from build123d import *

# Parameters (mm, degrees)
SKETCH1_W           = 70
SKETCH1_H           = 25
SKETCH1_R           = 1.6
BOSS_EXTRUDE1_DEPTH = 10
BOSS_EXTRUDE2_DEPTH = 25
SKETCH3_R           = 3
CUT_EXTRUDE1_DEPTH  = 39.487010796
FILLET1_R           = 2
SKETCH6_R           = 1.6
CUT_EXTRUDE3_DEPTH  = 27
SKETCH7_W           = 2.6
SKETCH7_H           = 6
CUT_EXTRUDE4_DEPTH  = 11.25


with BuildPart() as part:
    # Sketch1 → Boss-Extrude1 (new body)
    with BuildSketch(Plane(origin=(0, 0, 0), x_dir=(1, 0, 0), z_dir=(0, 1, 0))):
        Rectangle(SKETCH1_W, SKETCH1_H)
        with Locations(Location((-26, -1, 0), (0, 0, 270))):
            Circle(SKETCH1_R, mode=Mode.SUBTRACT)
        with Locations(Location((26, -1, 0), (0, 0, 270))):
            Circle(SKETCH1_R, mode=Mode.SUBTRACT)
    extrude(amount=BOSS_EXTRUDE1_DEPTH)

    # Sketch2 → Boss-Extrude2 (add)
    with BuildSketch(Plane.XY.offset(12.5)):
        Polygon((-35, 0), (-20.773502692, 0), (-15, -10), (-35, -10), align=None)
        Polygon((35, 0), (35, -10), (15, -10), (20.773502692, 0), align=None)
    extrude(amount=-BOSS_EXTRUDE2_DEPTH)

    # Sketch3 → Cut-Extrude1 (cut, through all)
    with BuildSketch(Plane.XZ):
        with Locations(Location((-26, 1, 0), (0, 0, 270))):
            Circle(SKETCH3_R)
        with Locations(Location((26, 1, 0), (0, 0, 270))):
            Circle(SKETCH3_R)
    extrude(amount=CUT_EXTRUDE1_DEPTH, mode=Mode.SUBTRACT)

    # Fillet1
    fillet1_edges = [part.edges().sort_by_distance(p)[0] for p in [
        (35, 10, 0),
        (0, 10, -12.5),
        (0, 0, -12.5),
        (0, 0, 12.5),
        (-17.886751346, -5, -12.5),
        (-25, -10, -12.5),
        (-15, -10, 0),
        (-25, -10, 12.5),
        (-17.886751346, -5, 12.5),
        (25, -10, -12.5),
        (17.886751346, -5, -12.5),
        (15, -10, 0),
        (25, -10, 12.5),
        (17.886751346, -5, 12.5),
        (-35, 10, 0),
        (-35, 0, -12.5),
        (35, 0, -12.5),
        (35, 0, 12.5),
        (-35, 0, 12.5),
        (0, 10, 12.5),
    ]]
    fillet(fillet1_edges, radius=FILLET1_R)

    # Sketch6 → Cut-Extrude3 (cut)
    with BuildSketch(Plane.ZY.offset(35)):
        with Locations((-8.5, -4)):
            Circle(SKETCH6_R)
        with Locations((7.5, -4)):
            Circle(SKETCH6_R)
    extrude(amount=-CUT_EXTRUDE3_DEPTH, mode=Mode.SUBTRACT)

    # Sketch7 → Cut-Extrude4 (cut)
    with BuildSketch(Plane.XZ.offset(10)):
        with Locations((-30, -8.5)):
            Rectangle(SKETCH7_W, SKETCH7_H)
        with Locations((-30, 7.5)):
            Rectangle(SKETCH7_W, SKETCH7_H)
    extrude(amount=-CUT_EXTRUDE4_DEPTH, mode=Mode.SUBTRACT)


solid = part.part
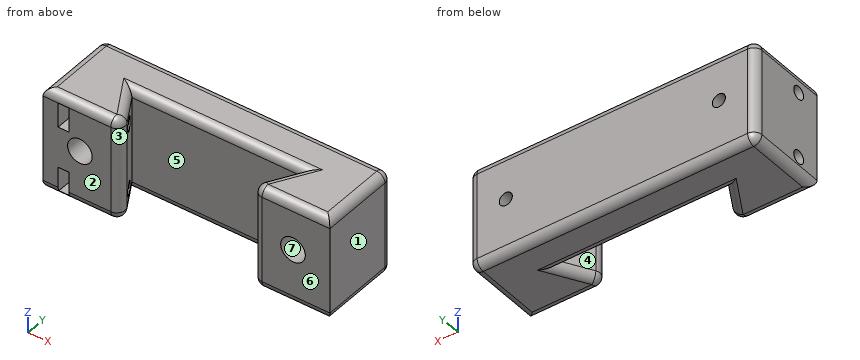
Can you work these out from the model? Positions are in its coordinate system, mm. Face numbers are marked on the shaded views. A direction names the side the tool comes from. Give positions to 0.01 mm unless a question says otherwise; leave off trailing zeros. Write each loop counter-clockwise with the first axis right and the second up, starting at its lowest first coordinate (ties: lowest second). Pieces come first, ordered by that corner, then holes. Notation, with made-up numbers: (53.5, 38) -> (95.5, 38) arc R8 cw to (95.5, 47) -> close; hole circle Ø3 at (25.25, 48). An arc over 180 degrees is marked (long way). Answer as a JSON object with one key per item and string values. Group by question number.
Item 1: I'm going to push flat-ended pins straight in: P1, Ø2, axis at x = -30, z = 6, coming from the -Y side; P2, Ø4, axis at x = 26, z = 1, coming from the -Y side; P3, Ø1.9, axis at y = -4, z = 7.5, coming from the -X side. Where does each tip first touch, or does it pass through?
Item 2: Please list where these lines run through material, in increasing order: line 1 (X direction, y = 4.5, z = 1); line 2 (Y direction, x = -32.65, z = -8.5); line 3 (X direction, y = -8.75, z = 9.5). Write a range as [from, to].
Item 3: Suppose I cut it at A-A (x = 26). Please give me the cut outline in (y, z), plus the area to 3 significant figures.
Item 4: For the marked faces 5, 6 and 7, which set-ups out of +Z, -Z, +X, -X, +Y, -Y let a thin tool reach every point of the face, with its end or its side?
Item 5: We'd pull the mould along Y, two halves only. Please class the marked faces 1, 2, 3 and 4: +Y half, -Y half, draft (parallel to the pull), parting line (faces both ways), or undercut.
Item 6: Suppose I cut it at D-D (x = -4.5). Please give me the cut outline in (y, z).
Item 7: Suppose I cut it at C-C (y = -4). State how many separate pieces and enclosed holes the cut face has, plus the area to 3 significant figures.
Item 8: Suppose I cut it at B-B (z = -8.5). Please give me the cut outline in (x, y).
Findings:
{
 "1": {"P1": "stops at y = 1.25", "P2": "stops at y = 0", "P3": "stops at x = 17.92"},
 "2": {"line 1": "x = [-35, -27.6], [-24.4, 24.4], [27.6, 35]", "line 2": "y = [-10, -5.6], [-2.4, 10]", "line 3": "x = [-35, -31.3], [-28.7, -16.61], [16.61, 35]"},
 "3": {"outline": "(-10, -10.5) arc R2 ccw to (-8, -12.5) -> (8, -12.5) arc R2 ccw to (10, -10.5) -> (10, -0.6) -> (0, -0.6) -> (0, -2) -> (-10, -2) -> close; (-10, 4) -> (0, 4) -> (0, 2.6) -> (10, 2.6) -> (10, 10.5) arc R2 ccw to (8, 12.5) -> (-8, 12.5) arc R2 ccw to (-10, 10.5) -> close", "area": "405 mm²"},
 "4": {"face 5": "+Z, -Z", "face 6": "+Z, -Z, +X, -X, -Y", "face 7": "-Y"},
 "5": {"face 1": "draft", "face 2": "-Y half", "face 3": "undercut", "face 4": "undercut"},
 "6": {"outline": "(0, -10.5) arc R2 ccw to (2, -12.5) -> (8, -12.5) arc R2 ccw to (10, -10.5) -> (10, 10.5) arc R2 ccw to (8, 12.5) -> (2, 12.5) arc R2 ccw to (0, 10.5) -> close"},
 "7": {"separate pieces": "4", "enclosed holes": "2", "area": "642 mm²"},
 "8": {"outline": "(-35, -10) -> (-31.3, -10) -> (-31.3, -5.6) -> (-35, -5.6) -> close; (-35, -2.4) -> (-31.3, -2.4) -> (-31.3, 1.25) -> (-28.7, 1.25) -> (-28.7, -2.4) -> (-19.39, -2.4) -> (-20.77, 0) -> (20.77, 0) -> (16.73, -7) arc R2 ccw to (18.46, -10) -> (35, -10) -> (35, 8) arc R2 ccw to (33, 10) -> (-33, 10) arc R2 ccw to (-35, 8) -> close; (-28.7, -10) -> (-18.46, -10) arc R2 ccw to (-16.73, -7) -> (-17.54, -5.6) -> (-28.7, -5.6) -> close"}
}
